Geometry check sheet. Reference: the model listing, model coordinates, mm. Face numbers are marked on the shaded views. Round coordinates to 2 decimals unless told otherwise and drop trailing zeros. Write each loop counter-clockwise with the first axis right and the second up, starting at its lowest first coordinate (ties: lowest second). Pieces come first, ordered by that corner, then holes. Notation, with made-up numbers: (-2, -38.75) -> (45, -38.75) arc R21 ccw to (45, -33.75) -> close; hole circle Ø1 at (31.5, 10). An arc over 180 degrees is marked (long way). Use a Markdown table: item, result.
```python
from build123d import *

# Parameters (mm, degrees)
F0_R     = 20.955
F1_DEPTH = 12.7
F2_R     = 19.2405
F3_DEPTH = 11.43
F4_R     = 1.27
F5_DEPTH = 2.54


with BuildPart() as f1:
    # F0 (on Top) → F1 (new body)
    with BuildSketch(Plane.XY):
        Circle(F0_R)
    extrude(amount=F1_DEPTH)

    # F2 (on face) → F3 (cut)
    with BuildSketch(Plane.XY.offset(12.7)):
        Circle(F2_R)
    extrude(amount=-F3_DEPTH, mode=Mode.SUBTRACT)

    # F4 (on face) → F5 (join)
    with BuildSketch(Plane(origin=(0, 0, 0), x_dir=(1, 0, 0), z_dir=(0, 0, -1))):
        with BuildLine():
            ThreePointArc((4.4199287209, 20.4835606061), (4.4387277549, 20.718947214), (4.445, 20.955))
            ThreePointArc((4.445, 20.955), (-0.236052786, 25.3937277549), (-4.4199287209, 20.4835606061))
            ThreePointArc((-4.4199287209, 20.4835606061), (0, 20.955), (4.4199287209, 20.4835606061))
        make_face()
        with Locations((0, 23.2695452869)):
            Circle(F4_R, mode=Mode.SUBTRACT)
    extrude(amount=-F5_DEPTH)


solid = f1.part
```
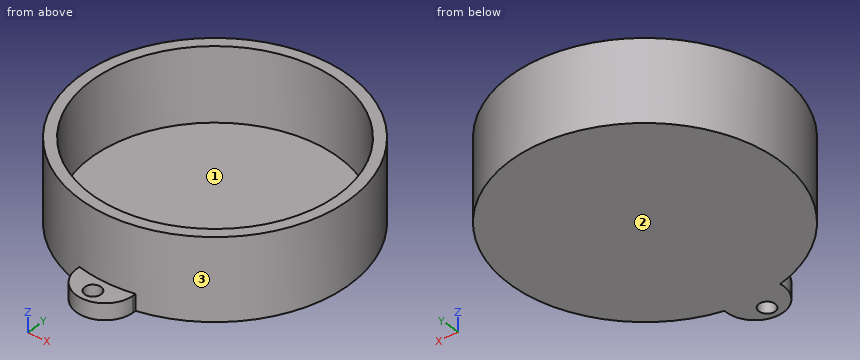
(1) Section check A-A on x = 0. Record the cut outline in (y, z) (1 decimal).
A:
| item | result |
|---|---|
| outline | (-25.4, 0) -> (-24.5, 0) -> (-24.5, 2.5) -> (-25.4, 2.5) -> close; (-22, 0) -> (21, 0) -> (21, 12.7) -> (19.2, 12.7) -> (19.2, 1.3) -> (-19.2, 1.3) -> (-19.2, 12.7) -> (-21, 12.7) -> (-21, 2.5) -> (-22, 2.5) -> close |
(2) Gauge pin test, flat ends, axial feed: pin 1 Ø4 at (x, y) = (2, -24) entering from +Z; pin 2 Ø19 at (x, y) = (-2.5, 0.5) entering from +Z; pin 3 Ø1.5 at (x, y) = (0, -23.27) entering from -Z; pin 4 Ø2 at (y, z) = (8.5, 3.5) entering from -X. Record the tip position at first contact, or that the pin passes through.
A:
| item | result |
|---|---|
| pin 1 | stops at z = 2.54 |
| pin 2 | stops at z = 1.27 |
| pin 3 | passes through |
| pin 4 | stops at x = -19.57 |
(3) Release check for a two-part mould opening along X. For the marked faces 1, 2 and 3 record: +X half, -X half, draft (parallel to the pull), parting line (faces both ways), or undercut.
A:
| item | result |
|---|---|
| face 1 | undercut |
| face 2 | draft |
| face 3 | parting line |
(4) Section check B-B on y = 0. Record the cut outline in (x, z) (1 decimal), plus the area to 3 significant figures.
A:
| item | result |
|---|---|
| outline | (-21, 0) -> (21, 0) -> (21, 12.7) -> (19.2, 12.7) -> (19.2, 1.3) -> (-19.2, 1.3) -> (-19.2, 12.7) -> (-21, 12.7) -> close |
| area | 92.4 mm2 |
(5) Section check C-C on z = 4. Record the cut outline in (x, y) (1 decimal), plus the area to 3 significant figures.
A:
| item | result |
|---|---|
| outline | circle Ø41.9 at (0, 0); hole circle Ø38.5 at (0, 0) |
| area | 217 mm2 |
(6) Thickness scan on line 1 (Y direction, x = 0, z = 2) (1 decimal); line 2 (Y direction, x = 0, z = 4.5) (1 decimal); line 3 (Y direction, x = 3, z = 11.75). Record the ranges inside material, lowest first.
A:
| item | result |
|---|---|
| line 1 | y = -25.4 to -24.5, -22 to -19.2, 19.2 to 21 |
| line 2 | y = -21 to -19.2, 19.2 to 21 |
| line 3 | y = -20.74 to -19.01, 19.01 to 20.74 |
(7) Section check D-D on x = 14. Record the cut outline in (y, z), plus the area to 3 significant figures.
A:
| item | result |
|---|---|
| outline | (-15.59, 0) -> (15.59, 0) -> (15.59, 12.7) -> (13.2, 12.7) -> (13.2, 1.27) -> (-13.2, 1.27) -> (-13.2, 12.7) -> (-15.59, 12.7) -> close |
| area | 94.3 mm2 |
